Can you work these out from the model? Positions are in its coordinate system, mm. Face numbers are marked on the shaded views. A direction names the side the tool comes from. Coordinates: 2 decimals unless noted, no trailing zeros. Write each loop counter-clockwise with the first axis right and the second up, starting at its lowest first coordinate (ties: lowest second). Pieces come first, ordered by that corner, then holes. Notation, with made-up numbers: (-14.75, 60.25) - (7.25, 60.25) arc R16 ccw to (7.25, 70.25) - close; hole circle Ø3 at (32.25, 43). An arc over 180 degrees is marked (long way). One line per question, with ' | ' between items. Start each with the question number.
from build123d import *

# Parameters (mm, degrees)
F0_W     = 250
F0_H     = 150
F1_DEPTH = 100
F2_W     = 220
F2_H     = 120
F3_DEPTH = 90
F4_R     = 20


with BuildPart() as f1:
    # F0 (on Top) → F1 (new body)
    with BuildSketch(Plane.XY):
        Rectangle(F0_W, F0_H)
    extrude(amount=F1_DEPTH)

    # F2 (on face) → F3 (cut)
    with BuildSketch(Plane.XY.offset(100)):
        with Locations((0, -1.488753)):
            Rectangle(F2_W, F2_H)
    extrude(amount=-F3_DEPTH, mode=Mode.SUBTRACT)

    # F4
    f4_edges = [f1.edges().sort_by_distance(p)[0] for p in [
        (125, -75, 50),
        (125, 75, 50),
        (-125, 75, 50),
        (-125, -75, 50),
    ]]
    fillet(f4_edges, radius=F4_R)


solid = f1.part
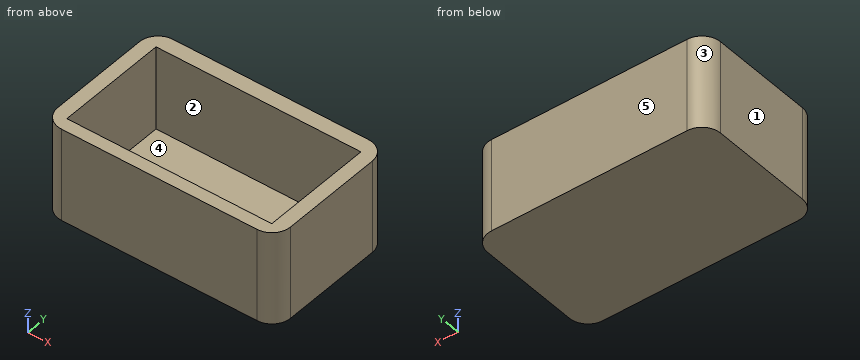
(1) Which directions (+Z, -Z, +X, -X, +Y, -Y) give clear straight access to the entire face, cutting with the end or side of a thin tool? Please do the marked faces 1 and 2.
(2) If we section it at C-C on x = 50.5: List the corners of the cut face in (y, z) for me, plus the area to 3 significant figures.
(3) I'm going to push a flat-ended pin straight in: pin 1 (1 mm diameter, centred on x = -21.5, y = -44, fed in from +Z). Where does the tip first touch, or does it pass through?
(4) If I drill on probe 1 along X at (y, z) = (13.5, 60); probe 2 along X at (y, z) = (-56.5, 62); probe 3 along Y at (x, z) = (100.5, 16.5), over which ranges is the centre line in solid material (lowest first)?
(5) If we section it at B-B on y = -9: List the corners of the cut face in (x, z) for me.
(6) If we section it at A-A on z = 45: List the corners of the cut face in (x, y) for me, plus the area to 3 significant figures.
(7) If we mould it in two halves opening along X, with no side actions, what happens to the marked faces 3, 4 and 5? For each: +X half, -X half, draft (parallel to the pull), parting line (faces both ways), or undercut.
Values:
1) face 1: +Z, -Z, -X, +Y, -Y | face 2: +Z
2) outline: (-75, 0) - (75, 0) - (75, 100) - (58.51, 100) - (58.51, 10) - (-61.49, 10) - (-61.49, 100) - (-75, 100) - close | area: 4,200 mm2
3) pin 1: z = 10
4) probe 1: -125 to -110, 110 to 125 | probe 2: -124.94 to -110, 110 to 124.94 | probe 3: -75 to -61.49, 58.51 to 75
5) outline: (-125, 0) - (125, 0) - (125, 100) - (110, 100) - (110, 10) - (-110, 10) - (-110, 100) - (-125, 100) - close
6) outline: (-125, -55) arc R20 ccw to (-105, -75) - (105, -75) arc R20 ccw to (125, -55) - (125, 55) arc R20 ccw to (105, 75) - (-105, 75) arc R20 ccw to (-125, 55) - close; hole (-110, -61.49) - (110, -61.49) - (110, 58.51) - (-110, 58.51) - close | area: 10,800 mm2
7) face 3: -X half | face 4: undercut | face 5: draft
